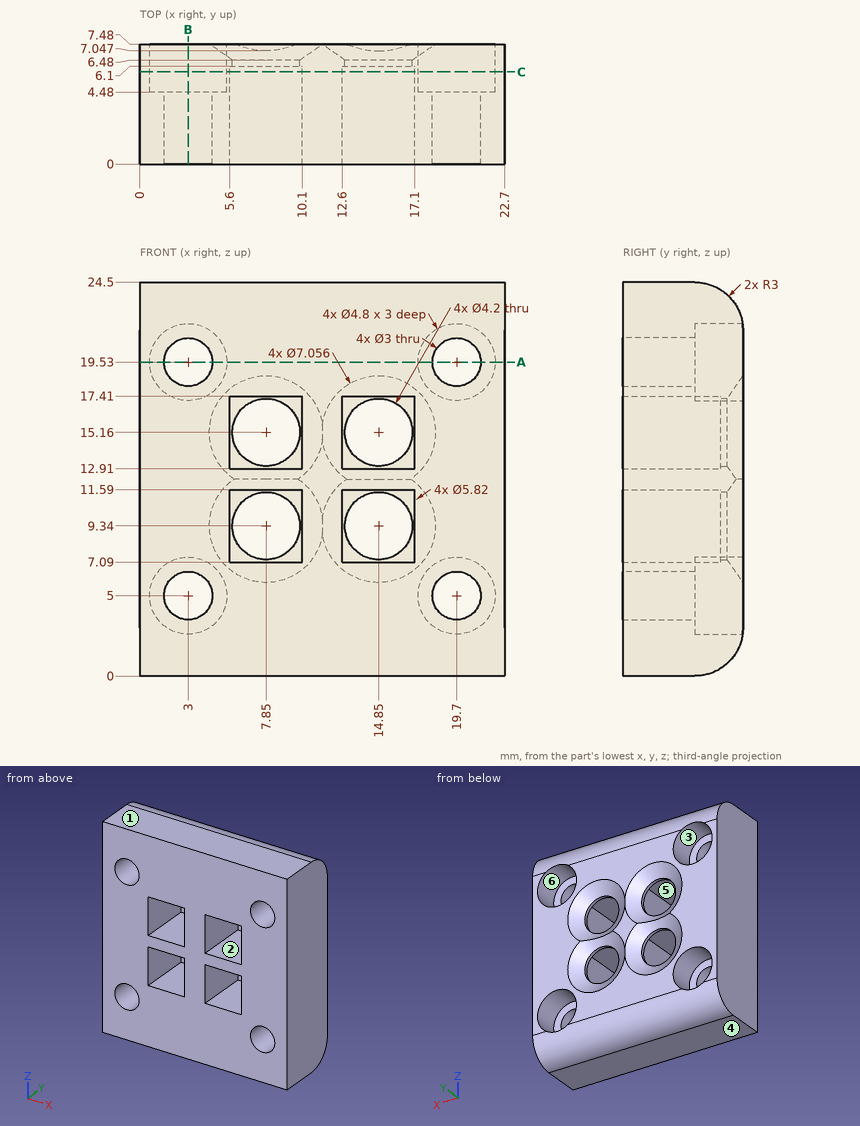
Job drawing, mm, ordinate dimensions from the low corner. One solid piece. A direction names the side the tool comes from. Coordinates: 2 decimals unless noted, no trailing zeros. Order: outer loops, then holes, each group sorted by start corner. A loop starts at its lowest first (then second) coordinate and runs counter-clockwise, first axis right, second up. Notation, with made-up numbers: M 46,-35.5 L 92,-35.5 A15 cw 92,-21.5 Z; hole C 82.5,58.5 d10. An arc over 180 degrees is marked long. Answer as CSV lines item,"result".
(1) Flat gauge pins, fed straight in: pin 1 (2.5 mm diameter, centred on x = 3, z = 4, fed in from +Y); pin 2 (1.5 mm diameter, centred on x = 8.5, z = 9.5, fed in from -Y); pin 3 (2 mm diameter, centred on x = 8, y = 6.5, fed in from +Z). Where does each tip first touch, or does it go through?
Geometry says:
pin 1,"stops at y = 4.48"
pin 2,"passes through"
pin 3,"stops at z = 24.32"
(2) Band-saw the part on A-A, the plane z = 19.53. List the corners of the cut face in (x, y), then the cut area to 3 significant figures.
Geometry says:
outline,"M 0,0 L 1.5,0 L 1.5,4.48 L 0.6,4.48 L 0.6,7.48 L 0,7.48 Z; M 4.5,0 L 18.2,0 L 18.2,4.48 L 17.3,4.48 L 17.3,7.48 L 5.4,7.48 L 5.4,4.48 L 4.5,4.48 Z; M 21.2,0 L 22.7,0 L 22.7,7.48 L 22.1,7.48 L 22.1,4.48 L 21.2,4.48 Z"
area,"114 mm2"
(3) Pull direction X, two halves, no side cores. Call the marked faces 1, 2 and 3: +X half, -X half, draft (parallel to the pull), parting line (faces both ways), or undercut.
Geometry says:
face 1,"draft"
face 2,"undercut"
face 3,"undercut"
(4) Band-saw the part on B-B, the plane x = 3. List the corners of the cut face in (y, z).
Geometry says:
outline,"M 0,0 L 4.48,0 A3 ccw 7.45,2.6 L 4.48,2.6 L 4.48,3.5 L 0,3.5 Z; M 0,6.5 L 4.48,6.5 L 4.48,7.4 L 7.48,7.4 L 7.48,17.13 L 4.48,17.13 L 4.48,18.03 L 0,18.03 Z; M 0,21.03 L 4.48,21.03 L 4.48,21.93 L 7.45,21.93 A3 ccw 4.48,24.5 L 0,24.5 Z"
(5) Band-saw the part on C-C, the plane y = 5.75. State how many separate pieces and enclosed holes the cut face has, then the cut area to 3 significant figures.
Geometry says:
separate pieces,"1"
enclosed holes,"8"
area,"390 mm2"
(6) 3-axis set-ups, long thin cutter, end or side, ignore diameter. For the marked faces 4, 5 and 6: which of +Z, -Z, +X, -X, +Y, -Y reach the whole face in a straight line?
Geometry says:
face 4,"-Z, +X, -X, +Y, -Y"
face 5,"-Y"
face 6,"+Y"
(7) Wall check: line 1 along X through (y, z) = (4.25, 9.5); line 2 along Z through (x, y) = (7, 4.5); line 3 along X through (y, z) = (1.95, 19.53). Give the ranges that are in metal, low to high.
Geometry says:
line 1,"x = 0 to 5.6, 10.1 to 12.6, 17.1 to 22.7"
line 2,"z = 0 to 7.09, 11.59 to 12.91, 17.41 to 24.5"
line 3,"x = 0 to 1.5, 4.5 to 18.2, 21.2 to 22.7"
